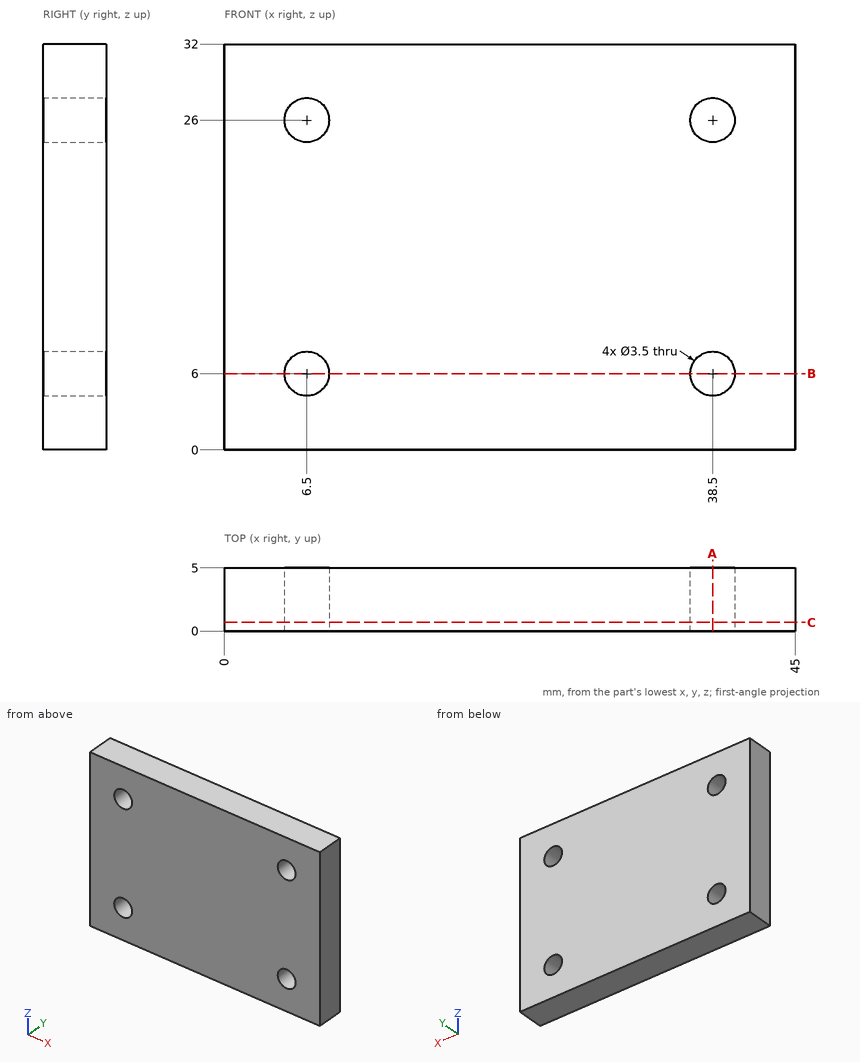
Check sheet for the drawn part. Datum: minimum x, y, z corner. Units: mm. Round coordinates to 2 decimals unless told otherwise and drop trailing zeros. Loops run counter-clockwise (first coordinate to the right, second up) from the corner with the lowest first, then second, coordinate; pieces in that order, holes last.
Item 1: Gauge pin test, flat end, axial feed: pin 1 (2 mm diameter, centred on x = 38.5, z = 26, fed in from -Y) (3 decimals). Record the tip position at first contact, or that the pin passes through.
Item 2: Thickness scan on line 1 (Z direction, x = 38.5, y = 2.9); line 2 (X direction, y = 2.3, z = 6); line 3 (Z direction, x = 37, y = 1.3). Record the ranges inside material, lowest first.
Item 3: Cross-section at B-B on z = 6. Record the boundary of the cut face in (x, y).
Item 4: Cross-section at C-C on y = 0.7. Record the boundary of the cut face in (x, z), then the cut area to 3 significant figures.
Item 5: Cross-section at A-A on x = 38.5. Record the boundary of the cut face in (y, z).
Answer sheet:
1. pin 1: passes through
2. line 1: z = 0 to 4.25, 7.75 to 24.25, 27.75 to 32
2. line 2: x = 0 to 4.75, 8.25 to 36.75, 40.25 to 45
2. line 3: z = 0 to 5.1, 6.9 to 25.1, 26.9 to 32
3. outline: (0, 0) - (4.75, 0) - (4.75, 5) - (0, 5) - close; (8.25, 0) - (36.75, 0) - (36.75, 5) - (8.25, 5) - close; (40.25, 0) - (45, 0) - (45, 5) - (40.25, 5) - close
4. outline: (0, 0) - (45, 0) - (45, 32) - (0, 32) - close; hole circle Ø3.5 at (6.5, 6); hole circle Ø3.5 at (6.5, 26); hole circle Ø3.5 at (38.5, 6); hole circle Ø3.5 at (38.5, 26)
4. area: 1,400 mm2
5. outline: (0, 0) - (5, 0) - (5, 4.25) - (0, 4.25) - close; (0, 7.75) - (5, 7.75) - (5, 24.25) - (0, 24.25) - close; (0, 27.75) - (5, 27.75) - (5, 32) - (0, 32) - close
